Part model, mm, in its own coordinate system. A direction names the side the tool comes from. Coordinates: 2 decimals unless noted, no trailing zeros. Order: outer loops, then holes, each group sorted by start corner. A loop starts at its lowest first (then second) coordinate and runs counter-clockwise, first axis right, second up.
1) Tool access for faces 1 (the flat face through (-5, -28, -11.9)), 2 (the flat face through (55, 66, 14.9)), 3 (the flat face through (-3.1, -28, 0)): list every direction of +Z, -Z, +X, -X, +Y, -Y with a clear straight run to the whole face (end or side of a thin tool).
2) Wall check: L1, parallel to Z at x = 56, y = 66; L2, parallel to Y at x = -4.1, z = 0; L3, parallel to Y at x = -4.05, z = 0. Give the ranges that are in metal, low to high.
3) Cut at C-C (y = -40). List the corners of the cut face in (x, z), and give its area (3 significant figures).
4) Mould opens along Z. For faces 4 (the flat face through (10, 39, -15)), 5 (the cylindrical face through (57.386, 59.779, -10.575)), 6 (the flat face through (55, 60, 14.9)), 7 (the cylindrical face through (-5.027, -41.464, -0.325)) say: +Z half, -Z half, draft (parallel to the pull), parting line (faces both ways), or undercut.
5) Pin check, flat tips, straight feed: pin 1 Ø1.9 at (x, y) = (-4.5, -40) entering from +Z; pin 2 Ø3 at (x, y) = (-4.5, -15) entering from -Z; pin 3 Ø2.5 at (x, y) = (57.5, 60) entering from +Z. Stop position of each tip, or through.
6) Cut at B-B (z = 0). List the corners of the cut face in (x, y).
7) Cut at D-D (z = -6). List the corners of the cut face in (x, y).
8) Cut at A-A (x = 53). List the corners of the cut face in (y, z).
```python
from build123d import *

# Parameters (mm, degrees)
BOSS_EXTRUDE1_DEPTH = 15
SKETCH2_W           = 3.8
SKETCH2_H           = 23.8
BOSS_EXTRUDE2_DEPTH = 56.9
SKETCH3_R           = 1.5
CUT_EXTRUDE1_DEPTH  = 3.8
SKETCH4_W           = 30
SKETCH4_H           = 3.8
SKETCH4_H_2         = 3
BOSS_EXTRUDE3_DEPTH = 13
CUT_EXTRUDE2_REACH  = 133.214
SKETCH5_R           = 1.5
SKETCH6_W           = 0.1
SKETCH6_H           = 10
CUT_EXTRUDE3_DEPTH  = 13


with BuildPart() as part:
    # Sketch1 → Boss-Extrude1 (new, symmetric)
    with BuildSketch(Plane.XY):
        with BuildLine():
            Line((-10, 0), (0, 0))
            ThreePointArc((0, 0), (11.925674657, 39.091125497), (48, 58.3))
            Line((48, 58.3), (48, 68.3))
            ThreePointArc((48, 68.3), (4.854606845, 46.162193309), (-10, 0))
        make_face()
    extrude(amount=BOSS_EXTRUDE1_DEPTH, both=True)

    # Sketch2 → Boss-Extrude2 (add)
    with BuildSketch(Plane.XZ):
        with Locations((-5, 0)):
            Rectangle(SKETCH2_W, SKETCH2_H)
    extrude(amount=BOSS_EXTRUDE2_DEPTH)

    # Sketch3 → Cut-Extrude1 (cut)
    with BuildSketch(Plane.ZY.offset(6.9)):
        with Locations((0, -20)):
            Circle(SKETCH3_R)
        with Locations((0, -40)):
            Circle(SKETCH3_R)
    extrude(amount=-CUT_EXTRUDE1_DEPTH, mode=Mode.SUBTRACT)

    # Sketch4 → Boss-Extrude3 (add)
    with BuildSketch(Plane(origin=(48, 0, 0), x_dir=(0, 0, -1), z_dir=(1, 0, 0))):
        with Locations((0, 66.4)):
            Rectangle(SKETCH4_W, SKETCH4_H)
        with Locations((0, 59.8)):
            Rectangle(SKETCH4_W, SKETCH4_H_2)
    extrude(amount=BOSS_EXTRUDE3_DEPTH)

    # Cut-Extrude2: up to this face of the body (flat: up to its plane)
    cut_extrude2_end = Plane(part.part.faces().sort_by_distance((54.5, 68.3, 0))[0])
    # Sketch5 → Cut-Extrude2 (cut, up to the picked face)
    with BuildSketch(Plane.XZ.offset(-58.3), mode=Mode.PRIVATE) as cut_extrude2_sk1:
        with Locations((56, 10)):
            Circle(SKETCH5_R)
    cut_extrude2_tool1 = split(extrude(cut_extrude2_sk1.sketch, amount=-CUT_EXTRUDE2_REACH, mode=Mode.PRIVATE), bisect_by=cut_extrude2_end, keep=Keep.BOTH, mode=Mode.PRIVATE)
    # Sketch5 → Cut-Extrude2 (cut, up to the picked face)
    with BuildSketch(Plane.XZ.offset(-58.3), mode=Mode.PRIVATE) as cut_extrude2_sk2:
        with Locations((56, -10)):
            Circle(SKETCH5_R)
    cut_extrude2_tool2 = split(extrude(cut_extrude2_sk2.sketch, amount=-CUT_EXTRUDE2_REACH, mode=Mode.PRIVATE), bisect_by=cut_extrude2_end, keep=Keep.BOTH, mode=Mode.PRIVATE)
    add(cut_extrude2_tool1.solids().sort_by(Axis((56, 58.3, 10), (0, 1, 0)))[0], mode=Mode.SUBTRACT)
    add(cut_extrude2_tool2.solids().sort_by(Axis((56, 58.3, -10), (0, 1, 0)))[0], mode=Mode.SUBTRACT)

    # Sketch6 → Cut-Extrude3 (cut)
    with BuildSketch(Plane(origin=(61, 0, 0), x_dir=(0, 0, -1), z_dir=(1, 0, 0))):
        with Locations((-14.95, 63.3)):
            Rectangle(SKETCH6_W, SKETCH6_H)
        with Locations((14.95, 63.3)):
            Rectangle(SKETCH6_W, SKETCH6_H)
    extrude(amount=-CUT_EXTRUDE3_DEPTH, mode=Mode.SUBTRACT)


solid = part.part
```
Geometry check:
1. face 1: -Z, +X, -X, -Y
1. face 2: +Z, +X, +Y, -Y
1. face 3: +Z, -Z, +X, -Y
2. L1: z = -14.9 to -11.5, -8.5 to 8.5, 11.5 to 14.9
2. L2: y = -56.9 to -41.5, -38.5 to -21.5, -18.5 to 32.3
2. L3: y = -56.9 to -41.5, -38.5 to -21.5, -18.5 to 32.4
3. outline: (-6.9, -11.9) - (-3.1, -11.9) - (-3.1, -1.5) - (-6.9, -1.5) - close; (-6.9, 1.5) - (-3.1, 1.5) - (-3.1, 11.9) - (-6.9, 11.9) - close
3. area: 79.0 mm2
4. face 4: -Z half
4. face 5: undercut
4. face 6: +Z half
4. face 7: undercut
5. pin 1: stops at z = 11.9
5. pin 2: stops at z = -11.9
5. pin 3: stops at z = 14.9
6. outline: (-10, 0) - (-6.9, 0) - (-6.9, -18.5) - (-3.1, -18.5) - (-3.1, 0) - (0, 0) arc R53.4 cw to (48, 58.3) - (61, 58.3) - (61, 61.3) - (48, 61.3) - (48, 64.5) - (61, 64.5) - (61, 68.3) - (48, 68.3) arc R63.36 ccw to start; (-6.9, -56.9) - (-3.1, -56.9) - (-3.1, -41.5) - (-6.9, -41.5) - close; (-6.9, -38.5) - (-3.1, -38.5) - (-3.1, -21.5) - (-6.9, -21.5) - close
7. outline: (-10, 0) - (-6.9, 0) - (-6.9, -56.9) - (-3.1, -56.9) - (-3.1, 0) - (0, 0) arc R53.4 cw to (48, 58.3) - (61, 58.3) - (61, 61.3) - (48, 61.3) - (48, 64.5) - (61, 64.5) - (61, 68.3) - (48, 68.3) arc R63.36 ccw to start
8. outline: (58.3, -14.9) - (61.3, -14.9) - (61.3, 14.9) - (58.3, 14.9) - close; (64.5, -14.9) - (68.3, -14.9) - (68.3, 14.9) - (64.5, 14.9) - close
